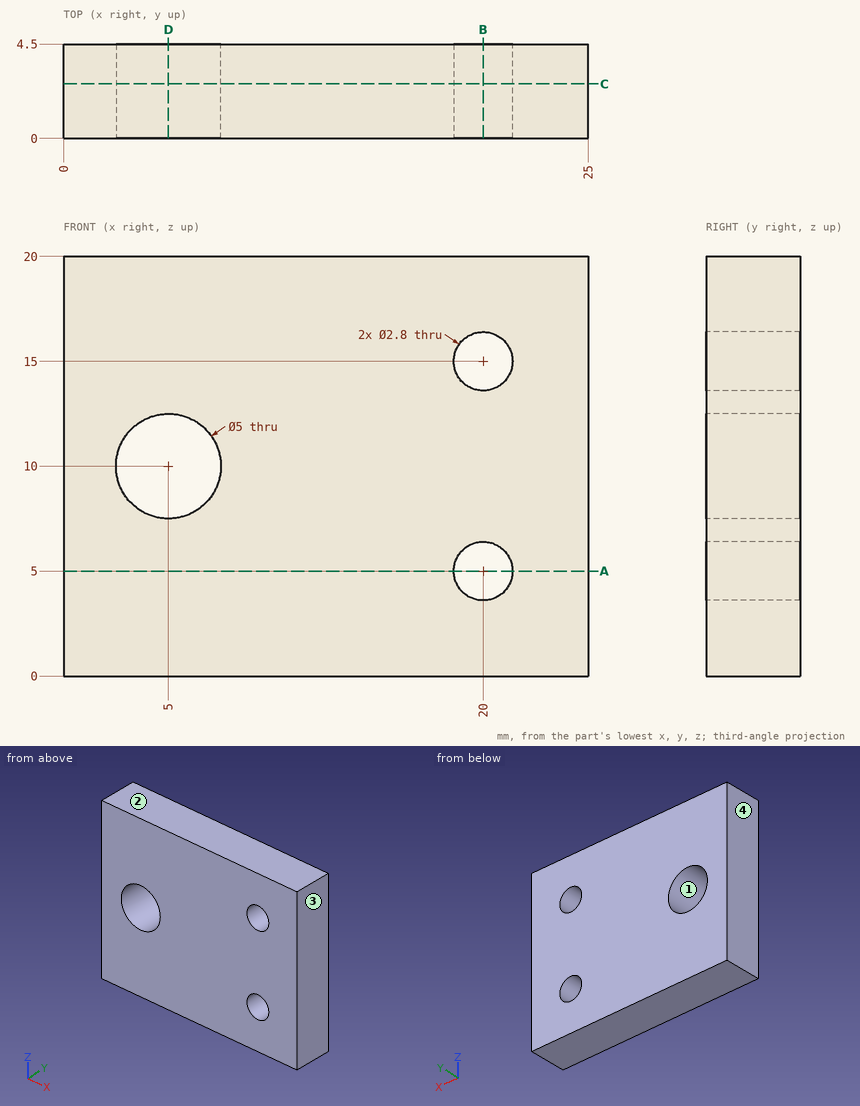
Check sheet for the drawn part. Datum: minimum x, y, z corner. Units: mm. Coordinates: 2 decimals unless noted, no trailing zeros. Order: outer loops, then holes, each group sorted by start corner. A loop starts at its lowest first (then second) coordinate and runs counter-clockwise, first axis right, second up. Notation, with made-up numbers: M 72.25,-39.75 L 97.25,-39.75 A26 ccw 97.25,-5.75 Z; hole C 29,6.25 d1. An arc over 180 degrees is marked long. One line per question, with ' | ' between items. Start each with the question number.
Item 1: Cross-section at A-A on z = 5. Enter the section's corners in (x, y).
Item 2: Cross-section at D-D on x = 5. Enter the section's corners in (y, z), then the cut area to 3 significant figures.
Item 3: Cross-section at C-C on y = 2.6. Enter the section's corners in (x, z), then the cut area to 3 significant figures.
Item 4: Gauge pin test, flat end, axial feed: pin 1 (3 mm diameter, centred on x = 5, z = 10, fed in from +Y). Record the tip position at first contact, or that the pin passes through.
Item 5: Draft check along X on the marked faces 1, 2, 3 and 4. Enter one of: pulls with the +X half, pulls with the -X half, needs draft (parallel to the pull), parting line crosses it, or undercut.
Item 6: Material ranges on L1, parallel to Z at x = 20, y = 1.5; L2, parallel to X at y = 2.6, z = 15; L3, parallel to X at y = 2.85, z = 10, recorded low to high. Write a range as [from, to].
Item 7: Cross-section at B-B on x = 20. Enter the section's corners in (y, z), then the cut area to 3 significant figures.
Findings:
1) outline: M 0,0 L 18.6,0 L 18.6,4.5 L 0,4.5 Z; M 21.4,0 L 25,0 L 25,4.5 L 21.4,4.5 Z
2) outline: M 0,0 L 4.5,0 L 4.5,7.5 L 0,7.5 Z; M 0,12.5 L 4.5,12.5 L 4.5,20 L 0,20 Z | area: 67.5 mm²
3) outline: M 0,0 L 25,0 L 25,20 L 0,20 Z; hole C 5,10 d5; hole C 20,5 d2.8; hole C 20,15 d2.8 | area: 468 mm²
4) pin 1: passes through
5) face 1: undercut | face 2: needs draft | face 3: pulls with the +X half | face 4: pulls with the -X half
6) L1: z = [0, 3.6], [6.4, 13.6], [16.4, 20] | L2: x = [0, 18.6], [21.4, 25] | L3: x = [0, 2.5], [7.5, 25]
7) outline: M 0,0 L 4.5,0 L 4.5,3.6 L 0,3.6 Z; M 0,6.4 L 4.5,6.4 L 4.5,13.6 L 0,13.6 Z; M 0,16.4 L 4.5,16.4 L 4.5,20 L 0,20 Z | area: 64.8 mm²
